For this review, take the finished solid that the model builds, in its own axes (mm). Face numbers are marked on the shaded views. A direction names the side the tool comes from. Round coordinates to 2 decimals unless told otherwise and drop trailing zeros. Write each loop counter-clockwise with the first axis right and the second up, starting at its lowest first coordinate (ties: lowest second). Pieces come first, ordered by that corner, then holes. Notation, with made-up numbers: (19.25, 78.5) -> (25.25, 78.5) arc R17 cw to (25.25, 97.5) -> close; hole circle Ø1 at (42, 74.25). An arc over 180 degrees is marked (long way). Answer as CSV lines item,"result". Start each with the question number.
Item 1: Wall thickness on probe 1 along X at (y, z) = (7, 7.5); probe 2 along Z at (x, y) = (105, 5); probe 3 along X at (y, z) = (5, 9.25): over which ranges is each line inside the solid? List them lowest first. Write a range as from..to.
Item 2: Take a section at B-B on z = 2.75. Give the boundary of the cut face in (x, y), then the cut area to 3 significant figures.
Item 3: For pin 1 Ø5.5 at (x, z) = (50, 6.5) entering from -Y; pin 2 Ø1.5 at (x, y) = (12, 10.5) entering from +Z; pin 3 Ø8 at (x, z) = (87, 13) entering from +Y; pin 4 Ø3.5 at (x, z) = (105, 7.5) entering from +Y, all flat-tipped, find the tip position at first contact; note any pin that passes through.
Item 4: Machinability: for the marked faces 1, 2 and 3, which of the approach directions +Z, -Z, +X, -X, +Y, -Y give a long, thin tool a straight path to every point of the face, cutting with its end or side? Answer none if there is none.
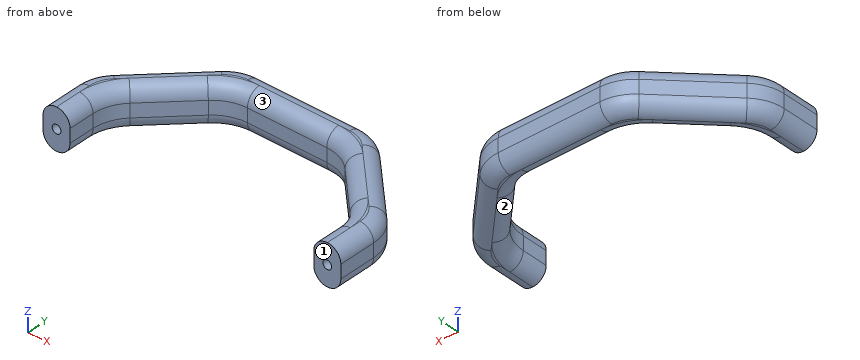
```python
from build123d import *

# Parameters (mm, degrees)
BOSS_EXTRU_1_DEPTH                  = 15
CONG_4_R                            = 15
CONG_5_R                            = 5
DIAM_TRE_DU_PER_AGE_3_2_3_2_1_D     = 3.2
DIAM_TRE_DU_PER_AGE_3_2_3_2_1_DEPTH = 10
DIAM_TRE_DU_PER_AGE_3_2_3_2_1_TIP   = 0.96137699


with BuildPart() as part:
    # Esquisse1 → Boss.-Extru.1 (new body)
    with BuildSketch(Plane.XY):
        Polygon((100, 0), (110, 0), (110, 20), (80, 50), (30, 50), (0, 20), (0, 0), (10, 0), (10, 15.857864376), (34.142135624, 40), (75.857864376, 40), (100, 15.857864376), align=None)
    extrude(amount=BOSS_EXTRU_1_DEPTH)

    # Congé4
    cong_4_edges = [part.edges().sort_by_distance(p)[0] for p in [
        (0, 20, 7.5),
        (30, 50, 7.5),
        (80, 50, 7.5),
        (110, 20, 7.5),
        (100, 15.857864376, 7.5),
        (75.857864376, 40, 7.5),
        (34.142135624, 40, 7.5),
        (10, 15.857864376, 7.5),
    ]]
    fillet(cong_4_edges, radius=CONG_4_R)

    # Congé5
    cong_5_edges = [part.edges().sort_by_distance(p)[0] for p in [
        (100, 4.82233047, 0),
        (98.858192988, 15.384912426, 0),
        (87.928932188, 27.928932188, 0),
        (75.384912426, 38.858192988, 0),
        (55, 40, 0),
        (34.615087574, 38.858192988, 0),
        (22.071067812, 27.928932188, 0),
        (11.141807012, 15.384912426, 0),
        (10, 4.82233047, 0),
        (0, 6.893398282, 0),
        (1.141807012, 19.52704805, 0),
        (15, 35, 0),
        (30.47295195, 48.858192988, 0),
        (55, 50, 0),
        (79.52704805, 48.858192988, 0),
        (95, 35, 0),
        (108.858192988, 19.52704805, 0),
        (110, 6.893398282, 0),
        (110, 6.893398282, 15),
        (108.858192988, 19.52704805, 15),
        (95, 35, 15),
        (79.52704805, 48.858192988, 15),
        (0, 6.893398282, 15),
        (1.141807012, 19.52704805, 15),
        (15, 35, 15),
        (30.47295195, 48.858192988, 15),
        (10, 4.82233047, 15),
        (11.141807012, 15.384912426, 15),
        (22.071067812, 27.928932188, 15),
        (34.615087574, 38.858192988, 15),
        (55, 40, 15),
        (75.384912426, 38.858192988, 15),
        (100, 4.82233047, 15),
        (98.858192988, 15.384912426, 15),
        (55, 50, 15),
        (87.928932188, 27.928932188, 15),
    ]]
    fillet(cong_5_edges, radius=CONG_5_R - 0.0001)  # a hair under: the kernel refuses the full size

    # Diamètre du perçage Ø3.2 (3.2)1
    with Locations(Plane(origin=(0, 0, 0), x_dir=(-1, 0, 0), z_dir=(0, -1, 0))):
        with Locations((-105, -7.5), (-5, -7.5)):
            Hole(DIAM_TRE_DU_PER_AGE_3_2_3_2_1_D / 2, depth=DIAM_TRE_DU_PER_AGE_3_2_3_2_1_DEPTH)
            with Locations((0, 0, -(DIAM_TRE_DU_PER_AGE_3_2_3_2_1_DEPTH + DIAM_TRE_DU_PER_AGE_3_2_3_2_1_TIP / 2))):  # 118° drill point
                Cone(0, DIAM_TRE_DU_PER_AGE_3_2_3_2_1_D / 2, DIAM_TRE_DU_PER_AGE_3_2_3_2_1_TIP, mode=Mode.SUBTRACT)


solid = part.part
```
Output values:
1,probe 1,"x = 0..3.4, 6.6..10, 100..103.4, 106.6..110"
1,probe 2,"z = 0..5.9, 9.1..15"
1,probe 3,"x = 0..10, 100..110"
2,outline,"(0.53, 0) -> (9.47, 0) -> (9.47, 9.64) arc R15.53 cw to (14.02, 20.63) -> (29.37, 35.98) arc R15.53 cw to (40.36, 40.53) -> (69.64, 40.53) arc R15.53 cw to (80.63, 35.98) -> (95.98, 20.63) arc R15.53 cw to (100.53, 9.64) -> (100.53, 0) -> (109.47, 0) -> (109.47, 13.79) arc R14.47 ccw to (105.23, 24.02) -> (84.02, 45.23) arc R14.47 ccw to (73.79, 49.47) -> (36.21, 49.47) arc R14.47 ccw to (25.98, 45.23) -> (4.77, 24.02) arc R14.47 ccw to (0.53, 13.79) -> close"
2,area,"1,420 mm^2"
3,pin 1,"stops at y = 40"
3,pin 2,"passes through"
3,pin 3,"stops at y = 46.31"
3,pin 4,"stops at y = 26.75"
4,face 1,"+Z, -Z, +X, -X, -Y"
4,face 2,"-Z, -Y"
4,face 3,"+Z, -Y"
